from build123d import *


with BuildPart() as part:
    # 草图1 → 旋转1 (revolve)
    with BuildSketch(Plane.XY, mode=Mode.PRIVATE) as revolve_1_sk:
        with BuildLine():
            Line((-4.3, 17), (-4.3, 13.5))
            ThreePointArc((-4.3, 13.5), (-3.762314929, 11.951026107), (-2.380543903, 11.068340325))
            Line((-2.380543903, 11.068340325), (0, 10.5))
            Line((0, 10.5), (-0.49797431, 10.00202569))
            Line((-0.49797431, 10.00202569), (-2.51987444, 10.484742003))
            ThreePointArc((-2.51987444, 10.484742003), (-4.233270511, 11.579272373), (-4.9, 13.5))
            Line((-4.9, 13.5), (-4.9, 17))
            Line((-4.9, 17), (-4.3, 17))
        make_face()
    revolve(revolve_1_sk.sketch.rotate(Axis((-48.745596361, 0, 0), (1, 0, 0)), 90), axis=Axis((-48.745596361, 0, 0), (1, 0, 0)))


solid = part.part
Geometry: final body of the model. Coordinates: model frame, mm. A direction names the side the tool comes from. Round coordinates to 2 decimals unless told otherwise and drop trailing zeros. Loops run counter-clockwise (first coordinate to the right, second up) from the corner with the lowest first, then second, coordinate; pieces in that order, holes last. Notation, with made-up numbers: M -19.5,69.5 L 37.5,69.5 A16 ccw 37.5,73.5 Z; hole C -15,37 d10. An arc over 180 degrees is marked long. One line per question, with ' | ' between items.
(1) Cut plane A-A on z = 0. Return the cut outline in (x, y).
Check result:
outline: M -4.9,-17 L -4.3,-17 L -4.3,-13.5 A2.5 cw -2.38,-11.07 L 0,-10.5 L -0.5,-10 L -2.52,-10.48 A3.1 ccw -4.9,-13.5 Z; M -4.9,13.5 A3.1 ccw -2.52,10.48 L -0.5,10 L 0,10.5 L -2.38,11.07 A2.5 cw -4.3,13.5 L -4.3,17 L -4.9,17 Z
(2) Material intervals for line 1 along Z through (x, y) = (-0.8, 9); line 2 along Z through (x, y) = (-3.5, -6); line 3 along Y through (x, z) = (-2.95, 8.5), sorted ascending. Write a range as from..to.
Check result:
line 1: z = -5.77..-4.53, 4.53..5.77 | line 2: z = -10.01..-9.11, 9.11..10.01 | line 3: y = -7.42..-6.37, 6.37..7.42
(3) Cut plane D-D on y = -14. Return the cut outline in (x, z).
Check result:
outline: M -4.9,-9.64 L -4.3,-9.64 L -4.3,9.64 L -4.9,9.64 Z
(4) Cut plane C-C on x = -1.9. Return the cut outline in (y, z).
Check result:
outline: C 0,0 d21.91; hole C 0,0 d20.67
(5) Access query for faces 1 (the flat face through (-4.3, -13, 5)), 2 (the flat face through (-4.9, -13, -5)). Directions: +Z, -Z, +X, -X, +Y, -Y. A direction counts if a zero-diameter tool reaches every point of the face in a straight line with its end or side. Return the directions, or none.
Check result:
face 1: +X | face 2: +Z, -Z, -X, +Y, -Y
(6) Contact query for flat-ended pins moving along their axis: P1, Ø1, axis at x = -0.5, y = -2, coming from the +Z side; P2, Ø2, axis at y = -10.5, z = 7.5, coming from the +X side. Output: stop coordinate, or through.
Check result:
P1: stops at z = 10.58 | P2: stops at x = -3.72
